The figure shows three views and two pictorial views of one solid part (mm, origin at its lowest corner). Answer the questions. A direction names the side the tool comes from. Coordinates: 2 decimals unless noted, no trailing zeros. Write each loop counter-clockwise with the first axis right and the second up, starting at its lowest first coordinate (ties: lowest second). Pieces come first, ordered by that corner, then holes. Notation, with made-up numbers: M -9.5,55 L -0.5,55 A28 ccw -0.5,77 Z; hole C -3.75,-27.5 d2. An arc over 180 degrees is marked long. Write item = value, one per line.
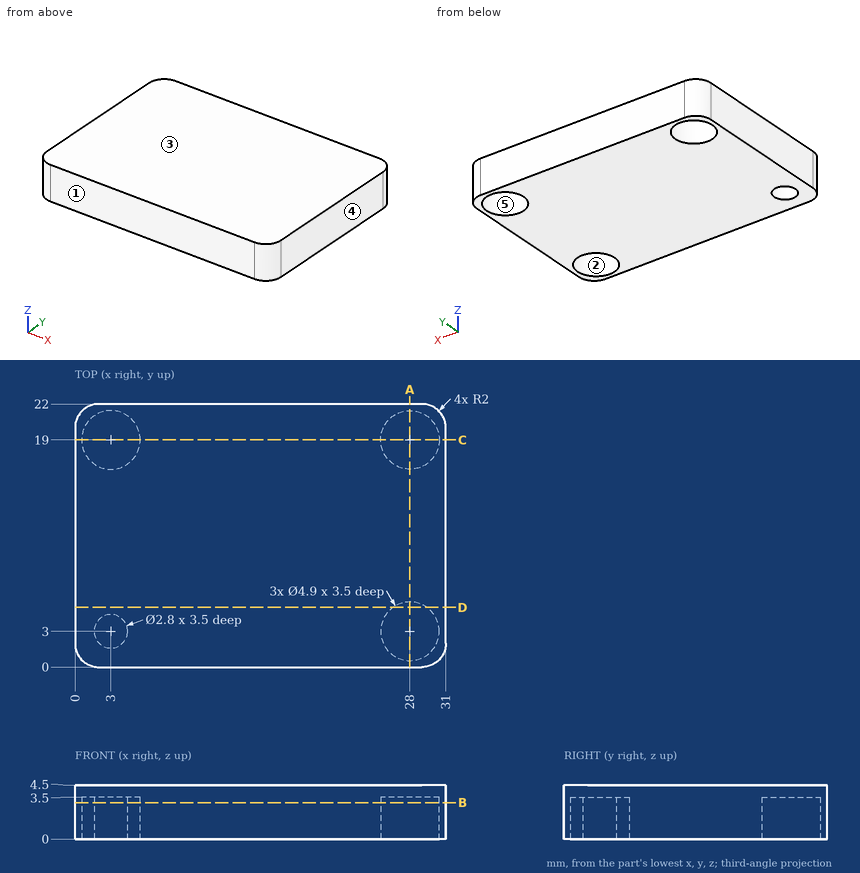
Item 1: Find section D-D (y = 5). Determine the outline of the cut face in (x, z), and give its area (3 significant figures).
Worked answers:
outline = M 0,0 L 26.58,0 L 26.58,3.5 L 29.42,3.5 L 29.42,0 L 31,0 L 31,4.5 L 0,4.5 Z
area = 130 mm²
Item 2: Find section A-A (x = 28). Determine the outline of the cut face in (y, z), and give its area (3 significant figures).
Worked answers:
outline = M 0,0 L 0.55,0 L 0.55,3.5 L 5.45,3.5 L 5.45,0 L 16.55,0 L 16.55,3.5 L 21.45,3.5 L 21.45,0 L 22,0 L 22,4.5 L 0,4.5 Z
area = 64.7 mm²
Item 3: A flat-ended cylindrical pin translates along its axis: pin 1 (2.5 mm diameter, centred on x = 27, y = 3.5, fed in from -Z). Find the tip coordinate at first contact, or state that the pin passes through.
Worked answers:
pin_1 = 3.5
Item 4: Consider line 1 along Y through (x, z) = (28, 1.4); line 2 along X through (y, z) = (3, 2.5); line 3 along X through (y, z) = (19, 1.4). Determine where each line is inside the solid, lowest interval first. Write a range as from..to.
Worked answers:
line_1 = 0..0.55, 5.45..16.55, 21.45..22
line_2 = 0..1.6, 4.4..25.55, 30.45..31
line_3 = 0..0.55, 5.45..25.55, 30.45..31
Item 5: Find section B-B (z = 3.05). Determine the outline of the cut face in (x, y), and give its area (3 significant figures).
Worked answers:
outline = M 0,2 A2 ccw 2,0 L 29,0 A2 ccw 31,2 L 31,20 A2 ccw 29,22 L 2,22 A2 ccw 0,20 Z; hole C 3,19 d4.9; hole C 3,3 d2.8; hole C 28,3 d4.9; hole C 28,19 d4.9
area = 616 mm²
Item 6: For a pull along X with two mould halves and no side action, classify the marked faces 3, 4 and 5 as released by +X, released by -X, zero draft, split by the parting line, or undercut.
Worked answers:
face_3 = zero draft
face_4 = released by +X
face_5 = undercut
Item 7: Find section C-C (y = 19). Determine the outline of the cut face in (x, z), and give its area (3 significant figures).
Worked answers:
outline = M 0,0 L 0.55,0 L 0.55,3.5 L 5.45,3.5 L 5.45,0 L 25.55,0 L 25.55,3.5 L 30.45,3.5 L 30.45,0 L 31,0 L 31,4.5 L 0,4.5 Z
area = 105 mm²
Item 8: Which of the six approach directions +Z, -Z, +X, -X, +Y, -Y give full straight-line access (tool end or side, diameter ignored) to the marked faces 1 and 2?
Worked answers:
face_1 = +Z, -Z, +X, -X, -Y
face_2 = -Z
